```python
from build123d import *

# Parameters (mm, degrees)
SKETCH_W        = 60
SKETCH_H        = 55
PAD_DEPTH       = 2.5
SKETCH001_W     = 2
SKETCH001_H     = 43
PAD001_DEPTH    = 30
SKETCH003_W     = 2
SKETCH003_H     = 43
PAD002_DEPTH    = 30
SKETCH004_W     = 1.5
SKETCH004_H     = 29.981854
PAD003_DEPTH    = 18.2
SKETCH005_W     = 1.5
SKETCH005_H     = 30
PAD004_DEPTH    = 18.2
SKETCH006_R     = 10.504142
POCKET_DEPTH    = 2
SKETCH007_W     = 0.78
SKETCH007_H     = 4.175734
POCKET001_DEPTH = 2
SKETCH009_R     = 8.511691
POCKET002_DEPTH = 2
SKETCH010_W     = 7.5
SKETCH010_H     = 16
POCKET003_DEPTH = 2
SKETCH011_W     = 14
SKETCH011_H     = 20
PAD005_DEPTH    = 9
SKETCH012_R     = 0.957136
SKETCH012_R_2   = 0.955296
POCKET004_DEPTH = 12


with BuildPart() as part:
    # Sketch → Pad (new body)
    with BuildSketch(Plane.YZ):
        with Locations((-4.822152, 15.702681)):
            Rectangle(SKETCH_W, SKETCH_H)
    extrude(amount=PAD_DEPTH)

    # Sketch001 (on Face6 of Pad) → Pad001 (join)
    with BuildSketch(Plane.YZ.offset(2.5)):
        with Locations((-31.822152, 15.702681)):
            Rectangle(SKETCH001_W, SKETCH001_H)
    extrude(amount=PAD001_DEPTH)

    # Sketch003 (on Face5 of Pad001) → Pad002 (join)
    with BuildSketch(Plane.YZ.offset(2.5)):
        with Locations((-11.722152, 15.702681)):
            Rectangle(SKETCH003_W, SKETCH003_H)
    extrude(amount=PAD002_DEPTH)

    # Sketch004 (on Face9 of Pad002) → Pad003 (join)
    with BuildSketch(Plane.ZX.offset(-30.822152)):
        with Locations((-5.047319, 17.509073)):
            Rectangle(SKETCH004_W, SKETCH004_H)
    extrude(amount=PAD003_DEPTH)

    # Sketch005 (on Face9 of Pad003) → Pad004 (join)
    with BuildSketch(Plane.ZX.offset(-30.822152)):
        with Locations((36.452681, 17.5)):
            Rectangle(SKETCH005_W, SKETCH005_H)
    extrude(amount=PAD004_DEPTH)

    # Sketch006 (on Face17 of Pad004) → Pocket (cut)
    with BuildSketch(Plane(origin=(0, -32.822152, 0), x_dir=(0, 0, -1), z_dir=(0, -1, 0))):
        with Locations((-20.702681, 17.5)):
            Circle(SKETCH006_R)
    extrude(amount=-POCKET_DEPTH, mode=Mode.SUBTRACT)

    # Sketch007 (on Face8 of Pocket) → Pocket001 (cut)
    with BuildSketch(Plane(origin=(0, 0, 37.202681), x_dir=(0, -1, 0), z_dir=(0, 0, 1))):
        with Locations((30.432152, 30.412133)):
            Rectangle(SKETCH007_W, SKETCH007_H)
    extrude(amount=-POCKET001_DEPTH, mode=Mode.SUBTRACT)

    # Sketch009 (on Face11 of Pocket) → Pocket002 (cut)
    with BuildSketch(Plane.ZX.offset(-10.722152)):
        with Locations((20.202681, 17.5)):
            Circle(SKETCH009_R)
    extrude(amount=-POCKET002_DEPTH, mode=Mode.SUBTRACT)

    # Sketch010 (on Face31 of Pocket002) → Pocket003 (cut)
    with BuildSketch(Plane.YX.offset(5.797319)):
        with Locations((-18.572152, 17.518146)):
            Rectangle(SKETCH010_W, SKETCH010_H)
    extrude(amount=-POCKET003_DEPTH, mode=Mode.SUBTRACT)

    # Sketch011 (on Face5 of Pocket003) → Pad005 (join)
    with BuildSketch(Plane.YZ.offset(2.5)):
        with Locations((6.277848, 20.002681)):
            Rectangle(SKETCH011_W, SKETCH011_H)
    extrude(amount=PAD005_DEPTH)

    # Sketch012 (on Face36 of Pad005) → Pocket004 (cut)
    with BuildSketch(Plane.YZ.offset(11.5)):
        with Locations((9.277848, 28.152681)):
            Circle(SKETCH012_R)
        with Locations((9.277848, 11.852681)):
            Circle(SKETCH012_R_2)
    extrude(amount=-POCKET004_DEPTH, mode=Mode.SUBTRACT)


solid = part.part
```
Here's how the part is built. I have some questions about the finished solid (model axes, mm). A direction names the side the tool comes from. Give positions to 0.01 mm unless a question says otherwise; leave off trailing zeros. Order: outer loops, then holes, each group sorted by start corner. A loop starts at its lowest first (then second) coordinate and runs counter-clockwise, first axis right, second up. Notation, with made-up numbers: M 39.25,25 L 84.25,25 A28 cw 84.25,56 Z; hole C 69.25,51.25 d5. An arc over 180 degrees is marked long. Use a Markdown table: item, result. Add a question column.
1. Suppose I cut it at A-A (y = -19.5). List the corners of the cut face in (x, z) for me, and give its area (3 significant figures).
2. Suppose I cut it at D-D (z = 25.5). List the corners of the cut face in (x, y) for me.
3. Suppose I cut it at B-B (x = 17.5). List the corners of the cut face in (y, z) for me, and give its area (3 significant figures).
4. I need wall thicknesses on probe 1 along Y at (x, z) = (6, 18.5); probe 2 along Z at (x, y) = (10, -24); probe 3 along Y at (x, z) = (11, 0.5). Which ranges of each line are inside material? Lowest first, please. Write a range as from..to.
5. If we mould it in two halves opening along Z, with no side actions, what happens to faces 6 (the flat face through (0, -5, 16)), 7 (the flat face through (17, -22, 37.203)), 8 (the cylindrical face through (8.18, -31.84, 15.86))? For each: +Z half, -Z half, draft (parallel to the pull), parting line (faces both ways), or undercut.
6. For pin 1 Ø4 at (x, z) = (12.5, 0.5) entering from +Y; pin 2 Ø6 at (y, z) = (-14.5, 18) entering from +X; pin 3 Ø4.5 at (x, y) = (7, 6.5) entering from -Z; pin 4 Ø1.6 at (x, z) = (21, -5) entering from -Y, each with a flat end and sliding along its axis, tell me the tip position at first contact or that it passes through.
7. Suppose I cut it at C-C (y = -26). List the corners of the cut face in (x, z) for me, and give its area (3 significant figures).
8. On a 3-axis mill with a long thin cutter (end or side, diameter ignored), from which of +Z, -Z, +X, -X, +Y, -Y can I reach the whole of each face in a straight line? I mean faces 1 (the flat face through (17, -22.322, -5)), 2 (the flat face through (7, 6, 10.003)), 3 (the flat face through (17, -10.722, 11)), 4 (the flat face through (7, 6, 30.003)), 5 (the flat face through (7, 13.278, 20)). Say none if no direction works.
Results list:
| question | item | result |
|---|---|---|
| 1 | outline | M 0,-11.8 L 2.5,-11.8 L 2.5,35.7 L 32.5,35.7 L 32.5,37.2 L 2.5,37.2 L 2.5,43.2 L 0,43.2 Z; M 2.52,-5.8 L 9.52,-5.8 L 9.52,-4.3 L 2.52,-4.3 Z; M 25.52,-5.8 L 32.5,-5.8 L 32.5,-4.3 L 25.52,-4.3 Z |
| 1 | area | 203 mm² |
| 2 | outline | M 0,-34.82 L 2.5,-34.82 L 2.5,-32.82 L 8.16,-32.82 L 8.16,-30.82 L 2.5,-30.82 L 2.5,-12.72 L 10.84,-12.72 L 10.84,-10.72 L 2.5,-10.72 L 2.5,-0.72 L 11.5,-0.72 L 11.5,13.28 L 2.5,13.28 L 2.5,25.18 L 0,25.18 Z; M 24.16,-12.72 L 32.5,-12.72 L 32.5,-10.72 L 24.16,-10.72 Z; M 26.84,-32.82 L 32.5,-32.82 L 32.5,-30.82 L 26.84,-30.82 Z |
| 3 | outline | M -32.82,-5.8 L -22.32,-5.8 L -22.32,-4.3 L -30.82,-4.3 L -30.82,10.2 L -32.82,10.2 Z; M -32.82,31.21 L -30.82,31.21 L -30.82,35.7 L -12.72,35.7 L -12.72,28.71 L -10.72,28.71 L -10.72,37.2 L -32.82,37.2 Z; M -14.82,-5.8 L -10.72,-5.8 L -10.72,11.69 L -12.72,11.69 L -12.72,-4.3 L -14.82,-4.3 Z |
| 3 | area | 139 mm² |
| 4 | probe 1 | y = -32.82..-30.82, -12.72..-10.72, -0.72..13.28 |
| 4 | probe 2 | z = -5.8..-4.3, 35.7..37.2 |
| 4 | probe 3 | y = -32.82..-30.82, -12.72..-10.72 |
| 5 | face 6 | draft |
| 5 | face 7 | +Z half |
| 5 | face 8 | undercut |
| 6 | pin 1 | stops at y = -10.72 |
| 6 | pin 2 | stops at x = 32.5 |
| 6 | pin 3 | stops at z = 10 |
| 6 | pin 4 | stops at y = -32.82 |
| 7 | outline | M 0,-11.8 L 2.5,-11.8 L 2.5,35.7 L 32.5,35.7 L 32.5,37.2 L 2.5,37.2 L 2.5,43.2 L 0,43.2 Z; M 2.52,-5.8 L 32.5,-5.8 L 32.5,-4.3 L 2.52,-4.3 Z |
| 7 | area | 227 mm² |
| 8 | face 1 | -Z |
| 8 | face 2 | -Z, +X, +Y |
| 8 | face 3 | +Z, -Z, +X |
| 8 | face 4 | +Z, +X, +Y |
| 8 | face 5 | +Z, -Z, +X, +Y |
